```python
from build123d import *

# Parameters (mm, degrees)
SM_BASE_FLANGE_1_DEPTH = 518


# Sheet-metal steps are written as plain solids
with BuildPart() as part:
    # Sketch 1 → Базовая кромка1 (new body)
    with BuildSketch(Plane.XY):
        with BuildLine():
            Line((-157.942286341, 0), (-128.947095812, 0))
            ThreePointArc((-128.947095812, 0), (-127.976524393, -0.127778151), (-127.072095812, -0.502404736))
            Line((-127.072095812, -0.502404736), (-50.174038106, -44.899519053))
            ThreePointArc((-50.174038106, -44.899519053), (-49.99315239, -44.97444437), (-49.799038106, -45))
            Line((-49.799038106, -45), (49.799038106, -45))
            ThreePointArc((49.799038106, -45), (49.99315239, -44.97444437), (50.174038106, -44.899519053))
            Line((50.174038106, -44.899519053), (127.072095812, -0.502404736))
            ThreePointArc((127.072095812, -0.502404736), (127.976524393, -0.127778151), (128.947095812, 0))
            Line((128.947095812, 0), (157.942286341, 0))
            Line((157.942286341, 0), (157.942286341, -3))
            Line((157.942286341, -3), (128.947095812, -3))
            ThreePointArc((128.947095812, -3), (128.752981528, -3.02555563), (128.572095812, -3.100480947))
            Line((128.572095812, -3.100480947), (51.674038106, -47.497595264))
            ThreePointArc((51.674038106, -47.497595264), (50.769609525, -47.872221849), (49.799038106, -48))
            Line((49.799038106, -48), (-49.799038106, -48))
            ThreePointArc((-49.799038106, -48), (-50.769609525, -47.872221849), (-51.674038106, -47.497595264))
            Line((-51.674038106, -47.497595264), (-128.572095812, -3.100480947))
            ThreePointArc((-128.572095812, -3.100480947), (-128.752981528, -3.02555563), (-128.947095812, -3))
            Line((-128.947095812, -3), (-157.942286341, -3))
            Line((-157.942286341, -3), (-157.942286341, 0))
        make_face()
    extrude(amount=SM_BASE_FLANGE_1_DEPTH)

    # Зеркальное отражение1: part across plane


with BuildPart() as part_1:
    add(part.part)
    add(part.part.mirror(Plane(origin=(51.674038106, -47.497595264, 0), x_dir=(1, 0, 0), z_dir=(0, 0, -1))))


solid = part_1.part
```
Part model, mm, in its own coordinate system. A direction names the side the tool comes from. Give positions to 0.01 mm unless a question says otherwise; leave off trailing zeros. Loops run counter-clockwise (first coordinate to the right, second up) from the corner with the lowest first, then second, coordinate; pieces in that order, holes last. Notation, with made-up numbers: M 25.5,24.25 L 84.5,24.25 A11 ccw 84.5,41.25 Z; hole C 24,-3 d7. An arc over 180 degrees is marked long. Return JSON: item names as keys, results as strings.
1) Saw through at D-D, the plane x = 73. List the corners of the cut face in (y, z), then the cut area to 3 significant figures.
Calculated:
{"outline": "M -35.19,-518 L -31.72,-518 L -31.72,518 L -35.19,518 Z", "area": "3,590 mm2"}
2) Saw through at A-A, the plane y = -10.5. List the corners of the cut face in (x, z).
Calculated:
{"outline": "M -115.76,-518 L -109.76,-518 L -109.76,518 L -115.76,518 Z; M 109.76,-518 L 115.76,-518 L 115.76,518 L 109.76,518 Z"}
3) Saw through at C-C, the plane x = 10.5. List the corners of the cut face in (y, z), then the cut area to 3 significant figures.
Calculated:
{"outline": "M -48,-518 L -45,-518 L -45,518 L -48,518 Z", "area": "3,110 mm2"}
4) Saw through at B-B, the plane z = -334. List the corners of the cut face in (x, y), then the cut area to 3 significant figures.
Calculated:
{"outline": "M -157.94,-3 L -128.95,-3 A0.75 cw -128.57,-3.1 L -51.67,-47.5 A3.75 ccw -49.8,-48 L 49.8,-48 A3.75 ccw 51.67,-47.5 L 128.57,-3.1 A0.75 cw 128.95,-3 L 157.94,-3 L 157.94,0 L 128.95,0 A3.75 ccw 127.07,-0.5 L 50.17,-44.9 A0.75 cw 49.8,-45 L -49.8,-45 A0.75 cw -50.17,-44.9 L -127.07,-0.5 A3.75 ccw -128.95,0 L -157.94,0 Z", "area": "1,020 mm2"}
5) Drill centre lines: line 1 (X direction, y = -17, z = 140.5); line 2 (X direction, y = -33.5, z = 235); line 3 (Y direction, x = -35.5, z = 118.5). Where is each one in solid material? Low to high.
Calculated:
{"line 1": "x = -104.5 to -98.5, 98.5 to 104.5", "line 2": "x = -75.92 to -69.92, 69.92 to 75.92", "line 3": "y = -48 to -45"}
6) 3-axis set-ups, long thin cutter, end or side, ignore diameter. For faces 4 (the face through (144, -3, 7)), 5 (the face through (-1, -45, 7)), 6 (the face through (-143, -3, 7)): which of +Z, -Z, +X, -X, +Y, -Y reach the whole face in a straight line?
Calculated:
{"face 4": "+Z, -Z, +X, -Y", "face 5": "+Z, -Z, +Y", "face 6": "+Z, -Z, -X, -Y"}
7) Flat gauge pins, fed straight in: pin 1 Ø14.5 at (x, z) = (146.5, 194) entering from -Y; pin 2 Ø10 at (x, z) = (109.5, -173) entering from +Y; pin 3 Ø2 at (y, z) = (-29, -400) entering from +X. Where does each tip first touch, or does it go through?
Calculated:
{"pin 1": "stops at y = -3", "pin 2": "stops at y = -7.76", "pin 3": "stops at x = 85.44"}
8) Pull direction X, two halves, no side cores. Call faces 1 (the face through (88.085, -23.012, 7.252)), 2 (the face through (143, 0, 7)), 3 (the face through (-89.6, -25.6, 7.3)): released by +X, released by -X, zero draft, split by the parting line, or undercut.
Calculated:
{"face 1": "undercut", "face 2": "zero draft", "face 3": "released by -X"}
